```python
from build123d import *

# Parameters (mm, degrees)
SKETCH1_R            = 5
BOSS_EXTRUDE1_DEPTH  = 10
FILLET1_DEPTH        = 10
FILLET1_2_DEPTH      = 10
M4_CLEARANCE_HOLE1_D = 4.5
FILLET2_R            = 5


with BuildPart() as part:
    # Sketch1 → Boss-Extrude1 (new body)
    with BuildSketch(Plane.XY):
        Polygon((10, -10), (45, -10), (45, -15), (-45, -15), (-45, -10), (-10, -10), (-10, 10), (10, 10), align=None)
        Circle(SKETCH1_R, mode=Mode.SUBTRACT)
    extrude(amount=BOSS_EXTRUDE1_DEPTH)

    # Fillet1: read off the stored shape, not the designer's step
    # Fillet1 outline → Fillet1 (cut)
    with BuildSketch(Plane.XY):
        with BuildLine():
            Line((10, 10), (0, 10))
            ThreePointArc((0, 10), (7.071067812, 7.071067812), (10, 0))
            Line((10, 0), (10, 10))
        make_face()
        with BuildLine():
            Line((-10, 10), (-10, 0))
            ThreePointArc((-10, 0), (-7.071067812, 7.071067812), (0, 10))
            Line((0, 10), (-10, 10))
        make_face()
    extrude(amount=FILLET1_DEPTH, mode=Mode.SUBTRACT)

    # Fillet1 2 outline → Fillet1 2 (add)
    with BuildSketch(Plane.XY):
        with BuildLine():
            ThreePointArc((20, -10), (12.928932188, -7.071067812), (10, 0))
            Line((10, 0), (10, -10))
            Line((10, -10), (20, -10))
        make_face()
        with BuildLine():
            ThreePointArc((-10, 0), (-12.928932188, -7.071067812), (-20, -10))
            Line((-20, -10), (-10, -10))
            Line((-10, -10), (-10, 0))
        make_face()
    extrude(amount=FILLET1_2_DEPTH)

    # M4 Clearance Hole1 (through all)
    with Locations(Plane(origin=(0, -10, 0), x_dir=(1, 0, 0), z_dir=(0, 1, 0))):
        with Locations((-35, -5), (35, -5)):
            Hole(M4_CLEARANCE_HOLE1_D / 2)

    # Fillet2
    fillet2_edges = [part.edges().sort_by_distance(p)[0] for p in [
        (45, -10, 5),
        (-45, -10, 5),
    ]]
    fillet(fillet2_edges, radius=FILLET2_R - 0.0001)  # a hair under: the kernel refuses the full size


solid = part.part
```
Input: part model. Units: mm. Frame: model coordinates. A direction names the side the tool comes from. Give positions to 0.01 mm unless a question says otherwise; leave off trailing zeros. Order: outer loops, then holes, each group sorted by start corner. A loop starts at its lowest first (then second) coordinate and runs counter-clockwise, first axis right, second up. Notation, with made-up numbers: (37, -15.5) - (82, -15.5) arc R14 ccw to (82, -9.5) - close; hole circle Ø9 at (-36.75, -37). An arc over 180 degrees is marked (long way). One line per item, written item: value.
1. Cut plane B-B, the plane z = 5. Give the number of separate pieces and of enclosed holes in the cut face, and give its area (3 significant figures).
Determined:
separate pieces: 3
enclosed holes: 1
area: 716 mm2
2. Draft query along X for faces 1 (the face through (0, -10, 0)), 2 (the face through (43, -11, 5)), 3 (the face through (-37.08, -12.53, 5.86)). Return one class per face: released by +X, released by -X, zero draft, split by the parting line, or undercut.
Determined:
face 1: zero draft
face 2: released by +X
face 3: undercut
3. Cut plane A-A, the plane x = -35. Output: boundary loops of the cut face in (y, z).
Determined:
outline: (-15, 0) - (-10, 0) - (-10, 2.75) - (-15, 2.75) - close; (-15, 7.25) - (-10, 7.25) - (-10, 10) - (-15, 10) - close
4. Line query: probe 1 along Z at (x, y) = (35, -11.55); probe 2 along Y at (x, z) = (34.5, 2.5); probe 3 along X at (y, z) = (-12, 3.75). Output: solid intervals per line, ascending.
Determined:
probe 1: 0 to 2.75, 7.25 to 10
probe 2: -15 to -10
probe 3: -44 to -36.87, -33.13 to 33.13, 36.87 to 44
5. Reachability of faces 4 (the face through (-30, -10, 5)), 5 (the face through (0, -10, 10)), 6 (the face through (30, -10, 5)) from +Z, -Z, +X, -X, +Y, -Y: full face, straight path, thin tool, end or side. Return the list, or none.
Determined:
face 4: +Z, -Z, -X, +Y
face 5: +Z, +X, -X, +Y, -Y
face 6: +Z, -Z, +X, +Y
6. Pin query (flat end, axial travel): pin 1 Ø6 at (x, z) = (35, 5) entering from -Y; pin 2 Ø1 at (y, z) = (-5.5, 4) entering from -X; pin 3 Ø1.5 at (x, z) = (-14, 4.5) entering from +Y; pin 4 Ø3 at (x, z) = (30.5, 5.5) entering from +Y. Return the tip coordinate at first contact, or that it passes through.
Determined:
pin 1: y = -15
pin 2: x = -12
pin 3: y = -7.38
pin 4: y = -10
7. Cut plane D-D, the plane y = 2.75. Output: boundary loops of the cut face in (x, z), and give its area (3 significant figures).
Determined:
outline: (-9.61, 0) - (-4.18, 0) - (-4.18, 10) - (-9.61, 10) - close; (4.18, 0) - (9.61, 0) - (9.61, 10) - (4.18, 10) - close
area: 109 mm2
